from build123d import *

# Parameters (mm, degrees)
BOSS_EXTRUDE1_DEPTH = 32


with BuildPart() as part:
    # Sketch1 → Boss-Extrude1 (new body)
    with BuildSketch(Plane(origin=(0, 0, 0), x_dir=(1, 0, 0), z_dir=(0, 1, 0))):
        with BuildLine():
            ThreePointArc((0, 64), (-32, 32), (0, 0))
            Line((0, 0), (0, 8))
            ThreePointArc((0, 8), (-24, 32), (0, 56))
            Line((0, 56), (0, 64))
        make_face()
        with BuildLine():
            Line((0, 8), (0, 0))
            ThreePointArc((0, 0), (22.627416998, 9.372583002), (32, 32))
            ThreePointArc((32, 32), (22.954114988, 54.295932479), (0.93071218, 63.986462368))
            Line((0.93071218, 63.986462368), (0, 64))
            Line((0, 64), (0, 56))
            ThreePointArc((0, 56), (16.970562748, 48.970562748), (24, 32))
            ThreePointArc((24, 32), (16.970562748, 15.029437252), (0, 8))
        make_face()
        with BuildLine():
            ThreePointArc((32, 32), (22.627416998, 9.372583002), (0, 0))
            Line((0, 0), (2200, 0))
            ThreePointArc((2200, 0), (2184, 16), (2200, 32))
            Line((2200, 32), (0.93071218, 63.986462368))
            ThreePointArc((0.93071218, 63.986462368), (22.954114988, 54.295932479), (32, 32))
        make_face()
        with BuildLine():
            ThreePointArc((2200, 32), (2184, 16), (2200, 0))
            Line((2200, 0), (2200, 32))
        make_face()
        with BuildLine():
            Line((2200, 32), (2200, 0))
            ThreePointArc((2200, 0), (2211.313708499, 4.686291501), (2216, 16))
            ThreePointArc((2216, 16), (2211.313708499, 27.313708499), (2200, 32))
        make_face()
    extrude(amount=BOSS_EXTRUDE1_DEPTH)


solid = part.part
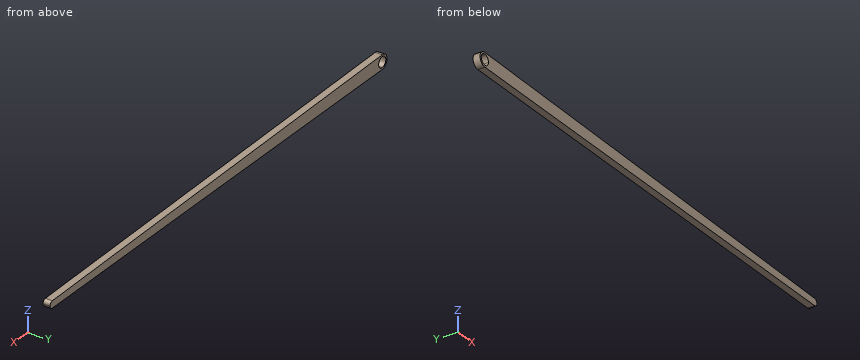
Check sheet for the modelled part. Datum: model origin and axes. Units: mm. Give positions to 0.01 mm unless a question says otherwise; leave off trailing zeros. Write each loop counter-clockwise with the first axis right and the second up, starting at its lowest first coordinate (ties: lowest second). Pieces come first, ordered by that corner, then holes. Notation, with made-up numbers: M 9.5,-29 L 44.5,-29 A28 ccw 44.5,-2 Z; hole C 56,-8.75 d7. An arc over 180 degrees is marked long. Use one line per item in the form item = value.
(1) Section check B-B on z = -43. Record the boundary of the cut face in (x, y), plus the area to 3 significant figures.
Answer block:
outline = M -30.05,0 L -21.33,0 L -21.33,32 L -30.05,32 Z; M 21.33,0 L 1443.75,0 L 1443.75,32 L 21.33,32 Z
area = 45,800 mm2
(2) Section check D-D on x = 440. Record the boundary of the cut face in (y, z), plus the area to 3 significant figures.
Answer block:
outline = M 0,-57.6 L 32,-57.6 L 32,0 L 0,0 Z
area = 1,840 mm2
(3) Material ranges on line 1 along X through (y, z) = (26, -25.5); line 2 along X through (y, z) = (13, -11); line 3 along Z through (x, y) = (430, 16), recorded low to high.
Answer block:
line_1 = -31.33 to -23.1, 23.1 to 2212.87
line_2 = -24.15 to -11.62, 11.62 to 2215.2
line_3 = -57.75 to 0
(4) Depth check by flat-ended pin: P1, Ø8, axis at y = 16.5, z = -31, coming from the -X side. Enter the tip coordinate at first touch or a pass-through.
Answer block:
P1 = -32
(5) Section check C-C on x = 1914. Record the boundary of the cut face in (y, z), plus the area to 3 significant figures.
Answer block:
outline = M 0,-36.16 L 32,-36.16 L 32,0 L 0,0 Z
area = 1,160 mm2
(6) Section check A-A on y = 17.5. Record the boundary of the cut face in (x, z), plus the area to 3 significant figures.
Answer block:
outline = M 0,-64 L 2200,-32 A16 ccw 2200,0 L 0,0 A32 ccw Z; hole C 0,-32 d48
area = 106,000 mm2
